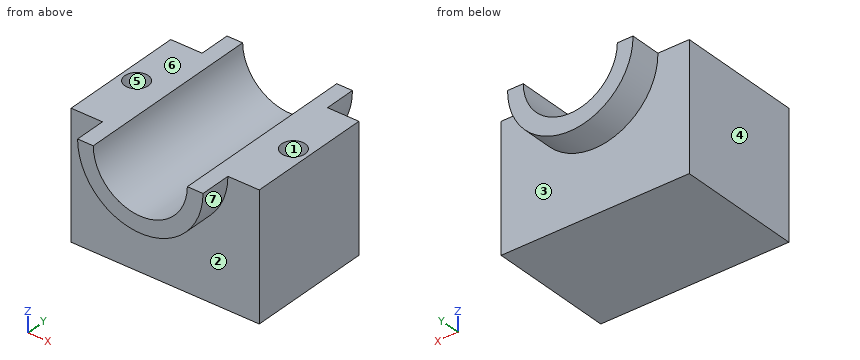
```python
from build123d import *

# Parameters (mm, degrees)
F0_W      = 152.4
F0_H      = 101.6
F1_DEPTH  = 101.6
F3_DEPTH  = 25.4
F4_DEPTH  = 128.27
F6_DEPTH  = 25.4
F7_R      = 9.525
F8_DEPTH  = 76.2
F9_R      = 9.525
F10_DEPTH = 76.2


with BuildPart() as f1:
    # F0 (on Top) → F1 (new body)
    with BuildSketch(Plane.XY):
        with Locations((2.3605413735, 24.3682915387)):
            Rectangle(F0_W, F0_H)
    extrude(amount=F1_DEPTH)

    # F2 (on face) → F3 (join)
    with BuildSketch(Plane.XZ.offset(26.4317084613)):
        with BuildLine():
            Line((-35.7394586265, 101.6), (-48.4394586265, 101.6))
            ThreePointArc((-48.4394586265, 101.6), (2.3605413735, 50.8), (53.1605413735, 101.6))
            Line((53.1605413735, 101.6), (40.4605413735, 101.6))
            ThreePointArc((40.4605413735, 101.6), (2.3605413735, 63.7227148693), (-35.7394586265, 101.6))
        make_face()
    extrude(amount=F3_DEPTH)

    # F4 (cut): a face of the model
    f4_faces = [f1.faces().sort_by_distance(p)[0] for p in [
        (2.3605413735, -26.4317084613, 85.532177983),
    ]]
    extrude(f4_faces, amount=-F4_DEPTH, mode=Mode.SUBTRACT)

    # F5 (on face) → F6 (join)
    with BuildSketch(Plane(origin=(0, 75.1682915387, 0), x_dir=(-1, 0, 0), z_dir=(0, 1, 0))):
        with BuildLine():
            Line((-40.4605413735, 101.6), (-53.1605413735, 101.6))
            ThreePointArc((-53.1605413735, 101.6), (-2.3605413735, 50.2605806131), (48.4394586265, 101.6))
            Line((48.4394586265, 101.6), (35.7394586265, 101.6))
            ThreePointArc((35.7394586265, 101.6), (-2.3605413735, 63.7227148693), (-40.4605413735, 101.6))
        make_face()
    extrude(amount=F6_DEPTH)

    # F7 (on face) → F8 (cut)
    with BuildSketch(Plane.XY.offset(101.6)):
        with Locations((-61.1394586265, 24.3682915387)):
            Circle(F7_R)
    extrude(amount=-F8_DEPTH, mode=Mode.SUBTRACT)

    # F9 (on face) → F10 (cut)
    with BuildSketch(Plane.XY.offset(101.6)):
        with Locations((65.8605413735, 24.3682915387)):
            Circle(F9_R)
    extrude(amount=-F10_DEPTH, mode=Mode.SUBTRACT)


solid = f1.part
```
The listing builds one solid part. Answer for the finished solid, in the listing's coordinates (mm). Face numbers are marked on the shaded views. A direction names the side the tool comes from. Coordinates: 2 decimals unless noted, no trailing zeros. Write each loop counter-clockwise with the first axis right and the second up, starting at its lowest first coordinate (ties: lowest second). Pieces come first, ordered by that corner, then holes. Notation, with made-up numbers: (-4.5, 80.25) - (7.5, 80.25) arc R19 ccw to (7.5, 115.25) - close; hole circle Ø9 at (-33, 82). An arc over 180 degrees is marked (long way). Return JSON: item names as keys, results as strings. Group by question number.
1. A cutting plane is placed at A-A, the plane z = 85. Determine the outline of the cut face in (x, y) (3 decimals).
2. A cutting plane is placed at C-C, the plane x = -46. Determine the outline of the cut face in (y, z).
3. Straight lines are drawn through the part: L1, parallel to Y at x = -62, z = 53; L2, parallel to X at y = 20.5, z = 61.5; L3, parallel to X at y = 29.5, z = 72. For each, find the intervals that lie inside material, in ascending order.
4. Which of the six approach directions +Z, -Z, +X, -X, +Y, -Y give full straight-line access (tool end or side, diameter ignored) to the marked faces 1, 2, 3 and 4?
5. Determine the mould class of the marked faces 5, 6 and 7 for opening direction X: released by +X, released by -X, zero draft, split by the parting line, or undercut.
6. A cutting plane is placed at B-B, the plane z = 54. Determine the outline of the cut face in (x, y) (3 decimals).
7. Given pin 1 (3 mm diameter, centred on x = 36, y = 41, fed in from +Z); pin 2 (12 mm diameter, centred on x = -6, y = 4.5, fed in from +Z); pin 3 (1.5 mm diameter, centred on x = -4.5, z = 22, fed in from +Y), each flat-ended and moving along its own axis, determine where each tip first touches the part or whether it passes through.
Ans:
{
 "1": {"outline": "(-73.839, -26.432) - (-45.651, -26.432) - (-45.651, -51.832) - (-31.825, -51.832) - (-31.825, 100.568) - (-45.836, 100.568) - (-45.836, 75.168) - (-73.839, 75.168) - close; (36.546, -51.832) - (50.372, -51.832) - (50.372, -26.432) - (78.561, -26.432) - (78.561, 75.168) - (50.557, 75.168) - (50.557, 100.568) - (36.546, 100.568) - close; hole circle Ø19.05 at (-61.139, 24.368); hole circle Ø19.05 at (65.861, 24.368)"},
 "2": {"outline": "(-51.83, 86.05) - (-26.43, 86.05) - (-26.43, 0) - (75.17, 0) - (75.17, 85.5) - (100.57, 85.5) - (100.57, 101.6) - (-51.83, 101.6) - close"},
 "3": {"L1": "-26.43 to 14.88, 33.85 to 75.17", "L2": "-73.84 to -69.84, -52.44 to 57.16, 74.56 to 78.56", "L3": "-73.84 to -69.16, -53.12 to -21.35, 26.07 to 57.84, 73.88 to 78.56"},
 "4": {"face 1": "+Z", "face 2": "-Z, -Y", "face 3": "-Z, +Y", "face 4": "+Z, -Z, -X, +Y, -Y"},
 "5": {"face 5": "undercut", "face 6": "zero draft", "face 7": "split by the parting line"},
 "6": {"outline": "(-73.839, -26.432) - (-15.384, -26.432) - (-15.384, -51.832) - (20.105, -51.832) - (20.105, -26.432) - (78.561, -26.432) - (78.561, 75.168) - (21.491, 75.168) - (21.491, 100.568) - (-16.77, 100.568) - (-16.77, 75.168) - (-73.839, 75.168) - close; hole circle Ø19.05 at (-61.139, 24.368); hole circle Ø19.05 at (65.861, 24.368)"},
 "7": {"pin 1": "z = 87.1", "pin 2": "z = 66.53", "pin 3": "y = 75.17"}
}
